from build123d import *

# Parameters (mm, degrees)
SKETCH_1_R      = 7.1
EXTRUDE_1_DEPTH = 2
FILLET_1_R      = 1.5
SKETCH_2_R      = 4.5
EXTRUDE_2_DEPTH = 2
SKETCH_3_R      = 6
EXTRUDE_3_DEPTH = 10
SKETCH_4_R      = 0.75
EXTRUDE_4_DEPTH = 10
SKETCH_5_R      = 8
SKETCH_5_R_2    = 6
EXTRUDE_5_DEPTH = 5


with BuildPart() as part:
    # 草图1 → 拉伸1 (new body)
    with BuildSketch(Plane(origin=(0, 0, 0), x_dir=(1, 0, 0), z_dir=(0, 1, 0))):
        with Locations(Location((0, 0, 0), (0, 0, 270))):
            Circle(SKETCH_1_R)
    extrude(amount=EXTRUDE_1_DEPTH)

    # 圆角1
    fillet_1_edges = [part.edges().sort_by_distance(p)[0] for p in [
        (0, 2, -7.1),
    ]]
    fillet(fillet_1_edges, radius=FILLET_1_R)

    # 草图2 → 拉伸2 (add)
    with BuildSketch(Plane(origin=(0, 2, 0), x_dir=(-1, 0, 0), z_dir=(0, 1, 0))):
        with Locations(Location((0, 0, 0), (0, 0, 90))):
            Circle(SKETCH_2_R)
    extrude(amount=EXTRUDE_2_DEPTH)

    # 草图3 → 拉伸3 (add)
    with BuildSketch(Plane.XZ):
        with Locations(Location((0, 0, 0), (0, 0, 90))):
            Circle(SKETCH_3_R)
    extrude(amount=EXTRUDE_3_DEPTH)

    # 草图4 → 拉伸4 (add)
    with BuildSketch(Plane.XZ.offset(10)):
        with Locations(Location((0, -2.4, 0), (0, 0, 270))):
            Circle(SKETCH_4_R)
        with Locations(Location((0, 2.4, 0), (0, 0, 270))):
            Circle(SKETCH_4_R)
    extrude(amount=EXTRUDE_4_DEPTH)

    # 草图5 → 拉伸5 (add)
    with BuildSketch(Plane.XZ.offset(1)):
        with Locations(Location((0, 0, 0), (0, 0, 270))):
            Circle(SKETCH_5_R)
        with Locations(Location((0, 0, 0), (0, 0, 90))):
            Circle(SKETCH_5_R_2, mode=Mode.SUBTRACT)
    extrude(amount=EXTRUDE_5_DEPTH)


solid = part.part
Verification items for the finished model (mm, model axes). A direction names the side the tool comes from. Give positions to 0.01 mm unless a question says otherwise; leave off trailing zeros. Write each loop counter-clockwise with the first axis right and the second up, starting at its lowest first coordinate (ties: lowest second). Pieces come first, ordered by that corner, then holes.
(1) Material ranges on line 1 (Y direction, x = -6.5, z = 0.75); line 2 (Y direction, x = 3, z = -5.25); line 3 (Y direction, x = -4.5, z = -1.5), recorded low to high.
(2) Cross-section at D-D (y = -6.5). Enter the section's corners in (x, z), plus the area to 3 significant figures.
(3) Access from +Z, -Z, +X, -X, +Y, -Y to the whole of each face (thin tool, end or side, straight path). Record for faces 4 (the face through (1.352, 2.986, 4.292)), 5 (the face through (-1.802, -7.972, 5.723)), 6 (the face through (6, 0, -2)).
(4) Cross-section at B-B (y = -17.25). Enter the section's corners in (x, z).
(5) Gauge pin test, flat ends, axial feed: pin 1 (1 mm diameter, centred on x = 3, y = -1.5, fed in from +Z); pin 2 (6 mm diameter, centred on x = 2, y = 1.5, fed in from -Z); pin 3 (1 mm diameter, centred on y = -2, z = -5.5, fed in from -X) (3 decimals). Record the tip position at first contact, or that the pin passes through.
(6) Mould release check, pull along Y, two halves, no side actions. Record for faces 1 (the face through (-0.732, -14.93, 2.563)), 2 (the face through (-1.802, -0.493, 5.723)), 3 (the face through (0, -10, 0)): +Y half, -Y half, draft (parallel to the pull), parting line (faces both ways), or undercut.
(7) Cross-section at C-C (y = -2.5). Enter the section's corners in (x, z).
Worked out:
1. line 1: y = -6 to -1, 0 to 1.67
1. line 2: y = -6 to -1, 0 to 1.93
1. line 3: y = -10 to 2
2. outline: circle Ø12 at (0, 0)
2. area: 113 mm2
3. face 4: +Y
3. face 5: -Y
3. face 6: none
4. outline: circle Ø1.5 at (0, -2.4); circle Ø1.5 at (0, 2.4)
5. pin 1: stops at z = 7.6
5. pin 2: stops at z = -7.99
5. pin 3: stops at x = -6.245
6. face 1: draft
6. face 2: undercut
6. face 3: -Y half
7. outline: circle Ø16 at (0, 0)
